Input: part model. Units: mm. Frame: model coordinates. Face numbers are marked on the shaded views. A direction names the side the tool comes from. Give positions to 0.01 mm unless a question says otherwise; leave off trailing zeros. Write each loop counter-clockwise with the first axis right and the second up, starting at its lowest first coordinate (ties: lowest second). Pieces come first, ordered by that corner, then holes. Notation, with made-up numbers: (30.25, 87.25) -> (74.25, 87.25) arc R4 cw to (74.25, 92.25) -> close; hole circle Ø2 at (61, -39.75). An arc over 180 degrees is marked (long way). Return JSON: item names as keys, results as strings. Group by question number.
Item 1: Set-up query: the marked faces 1 and 2. Return all of +Z, -Z, +X, -X, +Y, -Y with unobstructed straight access to the full face (end or side cutting, diameter ignored); none if empty.
Item 2: Section A-A, the plane z = 6. Return loops of the section in (x, y).
Item 3: Pin query (flat end, axial travel): P1, Ø5, axis at x = 14.5, z = 1.5, coming from the -Y side. Return the tip coordinate at first contact, or that it passes through.
Item 4: Section C-C, the plane y = 12. Return loops of the section in (x, z), then the cut area to 3 significant figures.
Item 5: Section B-B, the plane x = 8.5. Return loops of the section in (y, z), then the cut area to 3 significant figures.
Item 6: Line query: line 1 (Y direction, x = 17.25, z = 0.75); line 2 (X direction, y = 5, z = 9); line 3 (X direction, y = 13.25, z = 5). Output: solid intervals per line, ascending. Write a range as [from, to].
Autodesk Inventor part; units mm, degrees
ref_plane "YZ Plane" through (0, 0, 0) normal (1, 0, 0) x (0, 1, 0)
ref_plane "XZ Plane" through (0, 0, 0) normal (0, 1, 0) x (-1, 0, 0)
ref_plane "XY Plane" through (0, 0, 0) normal (0, 0, 1) x (1, 0, 0)
sketch "Boceto1" plane through (0, 0, 0) normal (0, 0, 1) x (1, 0, 0)
  line L0 (0, 0) -> (0, 20)
  line L1 (0, 20) -> (20, 20)
  line L2 (20, 20) -> (20, 15)
  line L3 (20, 15) -> (5, 15)
  line L4 (5, 15) -> (5, 0)
  line L5 (5, 0) -> (0, 0)
  line L6 (0, 12.84) -> (-1.8, 12.84)
  line L7 (-1.8, 12.84) -> (-1.8, 15.5)
  line L8 (-1.8, 15.5) -> (-3.44, 15.5)
  line L9 (-3.44, 15.5) -> (-3.44, 4.5)
  line L10 (-3.44, 4.5) -> (-1.8, 4.5)
  line L11 (-1.8, 4.5) -> (-1.8, 7.16)
  line L12 (-1.8, 7.16) -> (0, 7.16)
  line L13 (0, 12.84) -> (0, 7.16)
  dimension "d0" = 20
  dimension "d1" = 20
  dimension "d2" = 5
  dimension "d3" = 5
  dimension "d7" = 11
  dimension "d8" = 1.8
  dimension "d9" = 1.64
  dimension "d10" = 5.68
  dimension "d11" = 2.66
  dimension "d12" = 2.66
  dimension "d13" = 7.16
  dimension "d14" = 7.16
extrude "Extrusión1" add sketch "Boceto1" along normal blind 10 contours L0 L1 L2 L3 L4 L5
chamfer "Chaflán1" distance 6 angle 45 1 edges at (5, 15, 5)
equation "\"d11\" = d12"
equation "\"d13\" = d14"
properties part number "Soporte_cajas" material "Plástico PC/ABS"
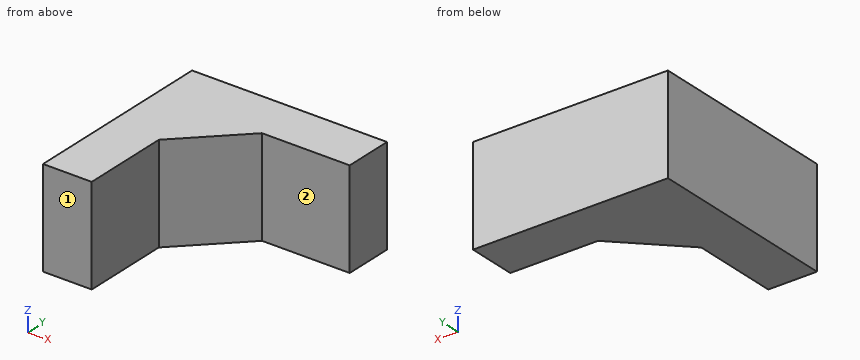
Answer below:
{
 "1": {"face 1": "+Z, -Z, +X, -X, -Y", "face 2": "+Z, -Z, +X, -Y"},
 "2": {"outline": "(0, 0) -> (5, 0) -> (5, 9) -> (11, 15) -> (20, 15) -> (20, 20) -> (0, 20) -> close"},
 "3": {"P1": "stops at y = 15"},
 "4": {"outline": "(0, 0) -> (8, 0) -> (8, 10) -> (0, 10) -> close", "area": "80.0 mm2"},
 "5": {"outline": "(12.5, 0) -> (20, 0) -> (20, 10) -> (12.5, 10) -> close", "area": "75.0 mm2"},
 "6": {"line 1": "y = [15, 20]", "line 2": "x = [0, 5]", "line 3": "x = [0, 9.25]"}
}
